CAD build for the part. Positions are in the model's coordinates, mm. A direction names the side the tool comes from. Coordinates: 2 decimals unless noted, no trailing zeros. Write each loop counter-clockwise with the first axis right and the second up, starting at its lowest first coordinate (ties: lowest second). Pieces come first, ordered by that corner, then holes. Notation, with made-up numbers: (85, -7) - (108, -7) arc R23 ccw to (108, 22) - close; hole circle Ø6 at (8, -5.5). An arc over 180 degrees is marked (long way). Answer in a Markdown table with one row per item. Add a question column.
Q1. Pin check, flat tips, straight feed: pin 1 (3.5 mm diameter, centred on x = -12, y = 12, fed in from -Z); pin 2 (10 mm diameter, centred on x = -18, z = -29.5, fed in from -Y); pin 3 (1.5 mm diameter, centred on x = -5, y = 16.5, fed in from +Z); pin 4 (1 mm diameter, centred on x = -20, y = 3, fed in from -Z). Stop position of each tip, or through.
Q2. Band-saw the part on D-D (z = -23). List the corners of the cut face in (x, y).
Q3. 3-axis set-ups, long thin cutter, end or side, ignore diameter. For faces 5 (the flat face through (-16, 7, 0)), 6 (the flat face through (-11, 9, -4.5)), 7 (the cylindrical face through (-21, 12, -18)): which of +Z, -Z, +X, -X, +Y, -Y reach the whole face in a straight line?
Q4. Two-plate mould, pull along Y, no slides. Class faces 1 (the cylindrical face through (-3, 12, -18)), 2 (the flat face through (-12, 1, -1)), 3 (the cylindrical face through (-12.89, 9.18, 3.63)), 4 (the flat face through (-12, 24, -3)): +Y half, -Y half, draft (parallel to the pull), parting line (faces both ways), or undercut.
Q5. Band-saw the part on B-B (z = -5.5). List the corners of the cut face in (x, y), and give its area (3 significant figures).
Q6. Drill centre lines: line 1 along X through (y, z) = (10.75, -7); line 2 along Y through (x, z) = (-21.55, -22.5); line 3 along Z through (x, y) = (-21.35, 12). Where is each one in solid material? Low to high. Write a range as from..to.
Q7. Band-saw the part on A-A (x = -12). List the corners of the cut face in (y, z), and give its area (3 significant figures).
Autodesk Inventor part; units mm, degrees
ref_plane "YZ Plane" through (0, 0, 0) normal (1, 0, 0) x (0, 1, 0)
ref_plane "XZ Plane" through (0, 0, 0) normal (0, 1, 0) x (-1, 0, 0)
ref_plane "XY Plane" through (0, 0, 0) normal (0, 0, 1) x (1, 0, 0)
sketch "Skizze1" plane through (0, 0, 0) normal (0, 1, 0) x (-1, 0, 0)
  line L0 (0, 0) -> (24, 0)
  line L1 (24, 0) -> (24, -34.5)
  line L2 (24, -34.5) -> (18, -34.5)
  line L3 (18, -34.5) -> (18, -4.5)
  line L4 (18, -4.5) -> (6, -4.5)
  line L5 (6, -4.5) -> (6, -34.5)
  line L6 (6, -34.5) -> (0, -34.5)
  line L7 (0, -34.5) -> (0, 0)
  dimension "d0" = 6
  dimension "d1" = 6
  dimension "d2" = 12
  dimension "d3" = 30
  dimension "d4" = 4.5
extrude "Extrusion1" add sketch "Skizze1" along normal blind 24
fillet "Rundung1" radius 12 2 edges at (-3, 24, -34.5) (-3, 0, -34.5)
fillet "Rundung2" radius 12 2 edges at (-21, 0, -34.5) (-21, 24, -34.5)
sketch "Skizze2" plane through (0, 0, 0) normal (1, 0, 0) x (0, 0, -1)
  arc A0 (22.5, 0) -> (22.5, 24) centre (22.5, 12) ccw
  point P0 (0, 0)
hole "Bohrung1" at (0, 12, -22.5) direction (-1, 0, 0) diameter 9 depth 24
chamfer "Fasen1" distance 2 angle 45 4 edges at (-12, 24, 0) (0, 12, 0) (-12, 0, 0) (-24, 12, 0)
sketch "Skizze3" plane through (-22, 2, 0) normal (0, 0, 1) x (1, 0, 0)
  circle A0 centre (10, 10) radius 6
  line L0 (-2, 22) -> (-2, -2)
  line L1 (0, 20) -> (20, 20)
  point P0 (22, -2)
  point P1 (-2, 10)
  point P2 (10, 20)
  dimension "d19" = 12
extrude "Extrusion2" add sketch "Skizze3" along normal blind 12
sketch "Skizze4" plane through (-12, 12, 12) normal (0, 0, 1) x (1, 0, 0)
  circle A0 centre (0, 0) radius 6
  point P0 (12, -12)
hole "Bohrung2" at (-12, 12, 12) direction (0, 0, -1) diameter 5.9175 depth 16.5 tip angle 118
properties part number "top_cylinder" material "Glasfaserbeton"
Checked values:
| question | item | result |
|---|---|---|
| 1 | pin 1 | passes through |
| 1 | pin 2 | stops at y = 0.17 |
| 1 | pin 3 | stops at z = 0 |
| 1 | pin 4 | stops at z = -30.97 |
| 2 | outline | (-24, 0.01) - (-18, 0.01) - (-18, 7.53) - (-24, 7.53) - close; (-24, 16.47) - (-18, 16.47) - (-18, 23.99) - (-24, 23.99) - close; (-6, 0.01) - (0, 0.01) - (0, 7.53) - (-6, 7.53) - close; (-6, 16.47) - (0, 16.47) - (0, 23.99) - (-6, 23.99) - close |
| 3 | face 5 | +Z |
| 3 | face 6 | -Z, +Y, -Y |
| 3 | face 7 | +X, -X |
| 4 | face 1 | undercut |
| 4 | face 2 | -Y half |
| 4 | face 3 | undercut |
| 4 | face 4 | +Y half |
| 5 | outline | (-24, 0) - (-18, 0) - (-18, 24) - (-24, 24) - close; (-6, 0) - (0, 0) - (0, 24) - (-6, 24) - close |
| 5 | area | 288 mm² |
| 6 | line 1 | x = -24..-18, -6..0 |
| 6 | line 2 | y = 0..7.5, 16.5..24 |
| 6 | line 3 | z = -34.5..-27, -18..0 |
| 7 | outline | (0, -4.5) - (9.04, -4.5) - (9.04, 12) - (6, 12) - (6, 0) - (2, 0) - (0, -2) - close; (14.96, -4.5) - (24, -4.5) - (24, -2) - (22, 0) - (18, 0) - (18, 12) - (14.96, 12) - close |
| 7 | area | 150 mm² |
